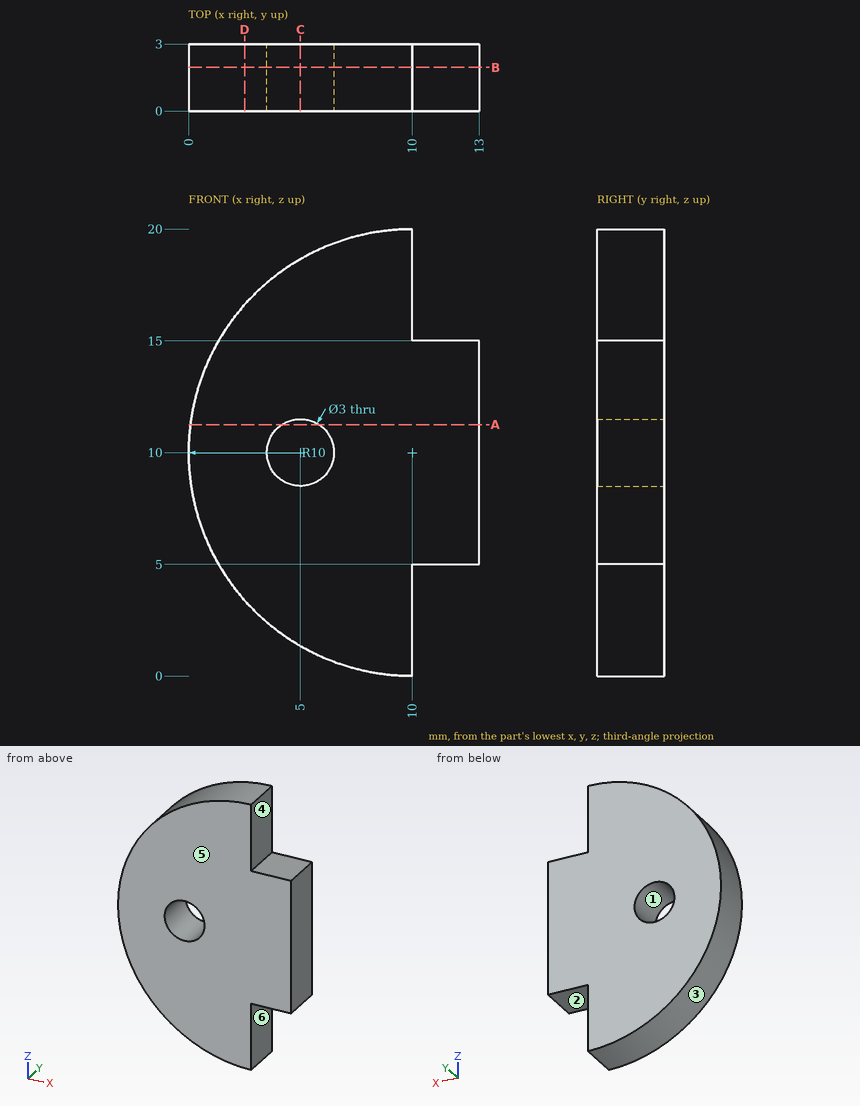
Geometry: see drawing. Coordinates: mm, zero at the bounding-box minimum. A direction names the side the tool comes from. Coordinates: 2 decimals unless noted, no trailing zeros. Loops run counter-clockwise (first coordinate to the right, second up) from the corner with the lowest first, then second, coordinate; pieces in that order, holes last. Notation, with made-up numbers: M -10,26 L 5,26 A28 ccw 5,55 Z; hole C 14,-26.75 d8. An arc over 180 degrees is marked long. Answer in a Markdown table with one row per item.
1. Reachability of the marked faces 4, 5 and 6 from +Z, -Z, +X, -X, +Y, -Y: full face, straight path, thin tool, end or side. Return the list, or none.
Response:
| item | result |
|---|---|
| face 4 | +Z, +X, +Y, -Y |
| face 5 | +Z, -Z, +X, -X, -Y |
| face 6 | -Z, +X, +Y, -Y |
2. Section C-C, the plane x = 5. Output: boundary loops of the cut face in (y, z), then the cut area to 3 significant figures.
Response:
| item | result |
|---|---|
| outline | M 0,1.34 L 3,1.34 L 3,8.5 L 0,8.5 Z; M 0,11.5 L 3,11.5 L 3,18.66 L 0,18.66 Z |
| area | 43.0 mm2 |
3. Draft query along X for the marked faces 1, 2 and 3. Return one class per face: pulls with the +X half, pulls with the -X half, needs draft (parallel to the pull), parting line crosses it, or undercut.
Response:
| item | result |
|---|---|
| face 1 | undercut |
| face 2 | needs draft |
| face 3 | pulls with the -X half |
4. Section B-B, the plane y = 1.95. Output: boundary loops of the cut face in (x, z), then the cut area to 3 significant figures.
Response:
| item | result |
|---|---|
| outline | M 10,0 L 10,5 L 13,5 L 13,15 L 10,15 L 10,20 A10 ccw Z; hole C 5,10 d3 |
| area | 180 mm2 |
5. Section A-A, the plane z = 11.25. Output: boundary loops of the cut face in (x, y).
Response:
| item | result |
|---|---|
| outline | M 0.08,0 L 4.17,0 L 4.17,3 L 0.08,3 Z; M 5.83,0 L 13,0 L 13,3 L 5.83,3 Z |
6. Material intervals for line 1 (X direction, y = 2.15, z = 10); line 2 (Z direction, x = 10.5, y = 2.45); line 3 (Z direction, x = 5, y = 1.25), sorted ascending.
Response:
| item | result |
|---|---|
| line 1 | x = 0 to 3.5, 6.5 to 13 |
| line 2 | z = 5 to 15 |
| line 3 | z = 1.34 to 8.5, 11.5 to 18.66 |
7. First-contact query: pin 1 (1.5 mm diameter, centred on y = 1, z = 3.5, fed in from +X); pin 2 (5 mm diameter, centred on x = 5, z = 10, fed in from +Y). Flat tips, straight axial feed; report the tip coordinate or a pass-through.
Response:
| item | result |
|---|---|
| pin 1 | stops at x = 10 |
| pin 2 | stops at y = 3 |
8. Section D-D, the plane x = 2.5. Output: boundary loops of the cut face in (y, z), then the cut area to 3 significant figures.
Response:
| item | result |
|---|---|
| outline | M 0,3.39 L 3,3.39 L 3,16.61 L 0,16.61 Z |
| area | 39.7 mm2 |
